Autodesk Inventor part; units mm, degrees
ref_plane "YZ Plane" through (0, 0, 0) normal (1, 0, 0) x (0, 1, 0)
ref_plane "XZ Plane" through (0, 0, 0) normal (0, 1, 0) x (-1, 0, 0)
ref_plane "XY Plane" through (0, 0, 0) normal (0, 0, 1) x (1, 0, 0)
ref_plane "Płaszczyzna konstrukcyjna1" through (-0.1106, 0.0064, 0) normal (0, 0, 1) x (1, 0, 0)
sketch "Szkic1" plane through (-0.1106, 0.0064, 0) normal (0, 0, 1) x (1, 0, 0)
  circle A0 centre (27.6196, -15.0064) radius 10
  circle A1 centre (27.6196, -15.0064) radius 10
  point P0 (0.1106, -0.0064)
  dimension "d0" = 20
extrude "Wyciągnięcie proste1" add sketch "Szkic1" along normal blind 180 and the other way blind 320
chamfer "Faza1" distance 2 angle 45 2 edges at (17.509, -15, 180) (17.509, -15, -320)
ref_plane "Płaszczyzna konstrukcyjna2" through (27.509, -15, -300) normal (0, 0, -1) x (-1, 0, 0)
sketch "Szkic2" plane through (27.509, -15, -300) normal (0, 0, -1) x (-1, 0, 0)
  circle A0 centre (0, 0) radius 10
  circle A1 centre (0, 0) radius 9
  point P0 (27.509, 15)
  dimension "d9" = 20
  dimension "d10" = 18
extrude "Wyciągnięcie proste2" cut sketch "Szkic2" against normal blind 2
pattern_linear "Szyk prostokątny1" count 24 spacing 20 along (0, 0, 1) of "Wyciągnięcie proste2"
properties part number "ryrka2"
The model under review builds one solid part; all positions refer to its coordinate system, in mm. A direction names the side the tool comes from. Give positions to 0.01 mm unless a question says otherwise; leave off trailing zeros. Write each loop counter-clockwise with the first axis right and the second up, starting at its lowest first coordinate (ties: lowest second). Pieces come first, ordered by that corner, then holes.
(1) To check wall thickness, follow L1, parallel to X at y = -14.25, z = -171.5; L2, parallel to X at y = -13.75, z = -234; L3, parallel to Y at x = 28, z = -201. State the ranges of each line that lie inside material, in increasing order.
(2) Consider section A-A, the plane z = -11.5. Give the boundary of the cut face in (x, y), and give its area (3 significant figures).
(3) Tool access review of faces 1 (the cylindrical face through (37.05, -18, 50.87)), 2 (the flat face through (36, -11, 40)): name each direction out of +Z, -Z, +X, -X, +Y, -Y from which nothing blocks a thin tool from reaching the whole face with its end or side.
(4) For P1, Ø12, axis at y = -12, z = -111, coming from the +X side; P2, Ø2, axis at x = 25.5, z = -37.5, coming from the -Y side; P3, Ø1.5, axis at x = 32, z = -76.5, coming from the +Y side, all flat-tipped, find the tip position at first contact; note any pin that passes through.
Returned:
1. L1: x = 17.54 to 37.48
1. L2: x = 17.59 to 37.43
1. L3: y = -24.99 to -5.01
2. outline: circle Ø20 at (27.51, -15)
2. area: 314 mm2
3. face 1: +Z, -Z
3. face 2: none
4. P1: stops at x = 37.51
4. P2: stops at y = -24.95
4. P3: stops at y = -5.73
